```python
from build123d import *

# Parameters (mm, degrees)
PAD020_DEPTH            = 6
THICKNESS_T             = -0.2
SKETCH043_W             = 0.1
SKETCH043_H             = 1
PAD001_DEPTH            = 1
SKETCH044_W             = 0.5
SKETCH044_H             = 0.5
PAD002_DEPTH            = 0.4
SKETCH003_W             = 0.32
SKETCH003_H             = 1.35
PAD003_DEPTH            = 0.1
BODY001_ROLL_ANGLE      = 90.000024
BODY001_PITCH_ANGLE     = -1e-05
BODY001_PLACEMENT_ANGLE = 45.000049


with BuildPart() as part:
    # Sketch042 → Pad020 (new body)
    with BuildSketch(Plane.XY):
        Polygon((0, 0), (6.5, 0), (7, -1), (6, -2.6), (0.5, -2.6), (-0.5, -1), align=None)
    extrude(amount=PAD020_DEPTH)

    # Thickness
    thickness_openings = [part.faces().sort_by_distance(p)[0] for p in [
        (3.25, -1.25728, 6),
    ]]
    offset(amount=THICKNESS_T, openings=thickness_openings)

    # Sketch043 (on Face5 of Thickness) → Pad001 (join)
    with BuildSketch(Plane.XZ.offset(2.6)):
        with Locations((5.95, 3)):
            Rectangle(SKETCH043_W, SKETCH043_H)
        with Locations((0.55, 3)):
            Rectangle(SKETCH043_W, SKETCH043_H)
    extrude(amount=PAD001_DEPTH)

    # Sketch044 (on Face7 of Pad001) → Pad002 (join)
    with BuildSketch(Plane.XZ.offset(2.6)):
        with Locations((1.35, 0.25)):
            Rectangle(SKETCH044_W, SKETCH044_H)
        with Locations((5.15, 0.25)):
            Rectangle(SKETCH044_W, SKETCH044_H)
    extrude(amount=PAD002_DEPTH)

    # Sketch003 (on Face7 of Pad002) → Pad003 (join)
    with BuildSketch(Plane.XZ.offset(2.6)):
        with Locations((1.81, -0.025)):
            Rectangle(SKETCH003_W, SKETCH003_H)
        with Locations((2.53, -0.025)):
            Rectangle(SKETCH003_W, SKETCH003_H)
        with Locations((3.25, -0.025)):
            Rectangle(SKETCH003_W, SKETCH003_H)
        with Locations((3.97, -0.025)):
            Rectangle(SKETCH003_W, SKETCH003_H)
        with Locations((4.69, -0.025)):
            Rectangle(SKETCH003_W, SKETCH003_H)
    extrude(amount=PAD003_DEPTH)


with BuildPart() as part_1:
    # Body001 roll: moved
    add(part.part.rotate(Axis((0, 0, 0), (1, 0, 0)), BODY001_ROLL_ANGLE))


with BuildPart() as part_2:
    # Body001 pitch: moved
    add(part_1.part.rotate(Axis((0, 0, 0), (0, 1, 0)), BODY001_PITCH_ANGLE))


with BuildPart() as part_3:
    # Body001 placement: moved
    add(part_2.part.moved(Location((37.1001, -41.6658, 24))).rotate(Axis((37.1001, -41.6658, 24), (0, 0, 1)), BODY001_PLACEMENT_ANGLE))


solid = part_3.part
```
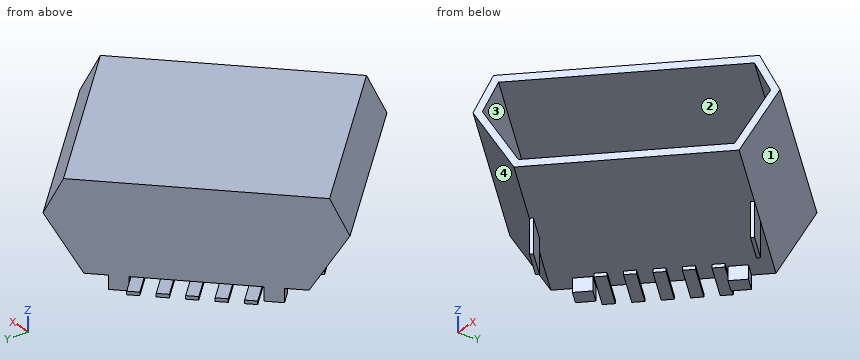
Geometry check sheet. Reference: the model listing, model coordinates, mm. Face numbers are marked on the shaded views. Give positions to 0.01 mm unless a question says otherwise; leave off trailing zeros. Order: outer loops, then holes, each group sorted by start corner. A loop starts at its lowest first (then second) coordinate and runs counter-clockwise, first axis right, second up.
1. Section check A-A, the plane y = -43.25. Enter the section's corners in (x, z), and give its area (3 significant figures).
2. Release check for a two-part mould opening along Y. For the marked faces 1, 2, 3 and 4 record: pulls with the +Y half, pulls with the -Y half, needs draft (parallel to the pull), parting line crosses it, or undercut.
3. Thickness scan on L1, parallel to Z at x = 42, y = -40.75; L2, parallel to X at y = -38.5, z = 23.45; L3, parallel to X at y = -39.5, z = 23.65. Record the ranges inside material, lowest first.
4. Section check D-D, the plane x = 43.25. Enter the section's corners in (y, z).
5. Section check B-B, the plane x = 45. Enter the section's corners in (y, z).
6. Gauge pin test, flat ends, axial feed: pin 1 Ø0.6 at (x, y) = (38.5, -39.5) entering from +Z; pin 2 Ø0.8 at (x, y) = (38, -40.5) entering from -Z; pin 3 Ø0.9 at (x, y) = (39, -39.5) entering from -Z; pin 4 Ø0.6 at (x, y) = (38.5, -40) entering from +Z. Record the tip position at first contact, or that the pin passes through.
7. Section check C-C, the plane z = 22.8. Enter the section's corners in (x, y), and give its area (3 significant figures).
Values follow:
1. outline: (37.98, 23) - (39.39, 21.4) - (39.39, 20.4) - (39.53, 20.4) - (39.53, 21.4) - (44, 21.4) - (44, 21.6) - (39.55, 21.6) - (38.3, 23.01) - (38.86, 23.8) - (44, 23.8) - (44, 24) - (38.68, 24) - close
1. area: 2.88 mm2
2. face 1: pulls with the +Y half
2. face 2: undercut
2. face 3: undercut
2. face 4: pulls with the -Y half
3. L1: z = 21.4 to 21.6, 23.8 to 24
3. L2: x = 40.27 to 40.55, 43.2 to 43.52
3. L3: x = 39.27 to 39.55, 44.06 to 44.37
4. outline: (-44, 21.4) - (-39.47, 21.4) - (-39.47, 20.4) - (-39.33, 20.4) - (-39.33, 21.4) - (-37.92, 23) - (-38.62, 24) - (-44, 24) - (-44, 23.8) - (-38.8, 23.8) - (-38.24, 23.01) - (-39.49, 21.6) - (-44, 21.6) - close
5. outline: (-42.25, 21.4) - (-41.08, 21.4) - (-39.67, 23) - (-40.37, 24) - (-42.25, 24) - (-42.25, 23.8) - (-40.55, 23.8) - (-39.99, 23.01) - (-41.24, 21.6) - (-42.25, 21.6) - close
6. pin 1: stops at z = 21.4
6. pin 2: stops at z = 21
6. pin 3: stops at z = 21.3
6. pin 4: stops at z = 24
7. outline: (36.83, -41.93) - (41.08, -46.17) - (41.24, -46.01) - (37.14, -41.91) - (41.94, -37.11) - (46.04, -41.21) - (46.2, -41.05) - (41.96, -36.8) - close
7. area: 4.19 mm2
